Autodesk Inventor part; units mm, degrees
ref_plane "YZ Plane" through (0, 0, 0) normal (1, 0, 0) x (0, 1, 0)
ref_plane "XZ Plane" through (0, 0, 0) normal (0, 1, 0) x (-1, 0, 0)
ref_plane "XY Plane" through (0, 0, 0) normal (0, 0, 1) x (1, 0, 0)
sketch "Sketch1" plane through (0, 0, 0) normal (0, 0, 1) x (1, 0, 0)
  line L0 (18.6296, 14.5185) -> (69.4296, 14.5185)
  line L1 (69.4296, 14.5185) -> (69.4296, 65.3185)
  line L2 (64.6696, 65.3185) -> (64.6696, 19.2785)
  line L3 (64.6696, 19.2785) -> (18.6296, 19.2785)
  line L4 (18.6296, 19.2785) -> (18.6296, 14.5185)
  line L5 (64.6696, 65.3185) -> (69.4296, 65.3185)
  point P0 (0, 0)
  dimension "d1" = 50.8
  dimension "d2" = 50.8
  dimension "d3" = 4.76
extrude "Extrusion1" add sketch "Sketch1" along normal blind 40
sketch "Sketch2" plane through (69.4296, 14.5185, 0) normal (1, 0, 0) x (0, 0, -1)
  line L0 (-40, 50.8) -> (0, 0)
  line L1 (-40, 0) -> (0, 50.0964)
  circle A0 centre (-20, 30.8) radius 12.5
  line L2 (0, 50.8) -> (-40, 50.8)
  line L3 (0, 0) -> (0, 50.8)
  point P0 (0, -14.5185)
  dimension "d6" = 25
  dimension "d7" = 20
  dimension "d8" = 20
extrude "Extrusion2" add sketch "Sketch2" against normal blind 19.76 contours A0 L1 L0 | L0 L1 A0 | L1 A0 L0 | L0 A0 L1
sketch "Sketch3" plane through (49.6696, 45.3185, 20) normal (-1, 0, 0) x (0, 0, 1)
  circle A0 centre (0, 0) radius 8
  point P0 (-20, -45.3185)
  dimension "d11" = 16
extrude "Extrusion3" cut sketch "Sketch3" against normal blind 19.76
sketch "Sketch4" plane through (18.6296, 14.5185, 0) normal (0, -1, 0) x (1, 0, 0)
  arc A0 (35.8, 15) -> (35.8, 25) centre (35.8, 20) ccw
  arc A1 (10, 25) -> (10, 15) centre (10, 20) ccw
  line L0 (50.8, 0) -> (50.8, 40)
  line L1 (0, 0) -> (0, 40)
  line L2 (0, 40) -> (50.8, 40)
  line L3 (35.8, 25) -> (10, 25)
  line L4 (10, 15) -> (35.8, 15)
  point P0 (-18.6296, 0)
  dimension "d14" = 10
  dimension "d15" = 10
  dimension "d16" = 15
  dimension "d17" = 10
  dimension "d18" = 20
  dimension "d19" = 20
extrude "Extrusion4" cut sketch "Sketch4" against normal blind 6
fillet "Fillet1" radius 2 1 edges at (69.4296, 14.5185, 20)
fillet "Fillet2" radius 2 2 edges at (67.0496, 65.3185, 40) (67.0496, 65.3185, 0)
sketch "Sketch5" plane through (18.6296, 19.2785, 0) normal (0, 1, 0) x (1, 0, 0)
  arc A0 (35.8, -25) -> (35.8, -15) centre (35.8, -20) ccw
  arc A1 (35.8, -25) -> (35.8, -15) centre (35.8, -20) ccw
  arc A2 (10, -15) -> (10, -25) centre (10, -20) ccw
  line L0 (10, -15) -> (35.8, -15)
  line L1 (35.8, -15) -> (10, -15)
  line L2 (35.8, -25) -> (10, -25)
  point P0 (-18.6296, 0)
equation "\"d19\" = d18"
properties part number "Mancal_Movel" material "SAE 1010/1020"
Part model, mm, in its own coordinate system. A direction names the side the tool comes from. Coordinates: 2 decimals unless noted, no trailing zeros. Write each loop counter-clockwise with the first axis right and the second up, starting at its lowest first coordinate (ties: lowest second). Pieces come first, ordered by that corner, then holes.
Item 1: Slice it at A-A (z = 20). Write the cut outline in (x, y).
Item 2: Which spindle directions (+Z, -Z, +X, -X, +Y, -Y) get a long thin tool onto all of the face, cutting with end or side? Do faces 4 (the face through (49.67, 37, 20)), 5 (the face through (57.275, 33.116, 22.71)), 6 (the face through (42, 17, 25)). Say none if no direction does.
Item 3: Slice it at D-D (y = 47.5). Write the cut outline in (x, z), and give its area (3 significant figures).
Item 4: Slice it at B-B (x = 31). Write the cut outline in (y, z).
Item 5: Mould opens along Y. For faces 1 (the face through (41, 17, 15)), 2 (the face through (42, 19.278, 11)), 3 (the face through (67.083, 64.717, 0.57)) say: released by +Y, released by -Y, zero draft, split by the parting line, or undercut.
Item 6: Probe line 1 (Y direction, x = 61, z = 20); line 2 (Y direction, x = 56.5, z = 20); line 3 (Z direction, x = 51, y = 17.5). List the from-to ranges inside material, lowest first.
Item 7: Slice it at C-C (y = 38.5). Write the cut outline in (x, z), and give its area (3 significant figures).
Item 8: Pin check, flat tips, straight feed: pin 1 (4 mm diameter, centred on x = 44, y = 17.5, fed in from -Z); pin 2 (20 mm diameter, centred on x = 42, z = 25.5, fed in from +Y); pin 3 (6 mm diameter, centred on x = 47.5, y = 37, fed in from -Z). Stop position of each tip, or through.
Results found:
1. outline: (18.63, 14.52) - (23.63, 14.52) - (23.63, 19.28) - (18.63, 19.28) - close; (49.67, 32.82) - (64.67, 32.82) - (64.67, 19.28) - (59.43, 19.28) - (59.43, 14.52) - (67.43, 14.52) arc R2 ccw to (69.43, 16.52) - (69.43, 37.32) - (49.67, 37.32) - close; (49.67, 53.32) - (69.43, 53.32) - (69.43, 65.32) - (64.67, 65.32) - (64.67, 57.82) - (49.67, 57.82) - close
2. face 4: +Z, -Z, -X, +Y
2. face 5: -X
2. face 6: -Y
3. outline: (49.67, 7.69) - (64.67, 7.69) - (64.67, 0) - (69.43, 0) - (69.43, 12.3) - (49.67, 12.3) - close; (49.67, 27.7) - (69.43, 27.7) - (69.43, 40) - (64.67, 40) - (64.67, 32.31) - (49.67, 32.31) - close
3. area: 255 mm2
4. outline: (14.52, 0) - (19.28, 0) - (19.28, 15) - (14.52, 15) - close; (14.52, 25) - (19.28, 25) - (19.28, 40) - (14.52, 40) - close
5. face 1: zero draft
5. face 2: undercut
5. face 3: released by +Y
6. line 1: y = 14.52 to 19.28, 32.82 to 37.32, 53.32 to 57.82
6. line 2: y = 32.82 to 37.32, 53.32 to 57.82
6. line 3: z = 0 to 15, 25 to 40
7. outline: (49.67, 9.52) - (64.67, 9.52) - (64.67, 0) - (69.43, 0) - (69.43, 15.82) - (49.67, 15.82) - close; (49.67, 24.18) - (69.43, 24.18) - (69.43, 40) - (64.67, 40) - (64.67, 30.48) - (49.67, 30.48) - close
7. area: 339 mm2
8. pin 1: stops at z = 0
8. pin 2: stops at y = 57.82
8. pin 3: stops at z = 9.17
